Source: three-view drawing plus pictorial views. Frame: mm from the lowest corner of the part. Round coordinates to 2 decimals unless told otherwise and drop trailing zeros. Write each loop counter-clockwise with the first axis right and the second up, starting at its lowest first coordinate (ties: lowest second). Pieces come first, ordered by that corner, then holes. Notation, with made-up numbers: (20, 44) -> (45, 44) arc R23 cw to (45, 75) -> close; hole circle Ø6 at (40.25, 70). An arc over 180 degrees is marked (long way). Put each result on its own line as item: value.
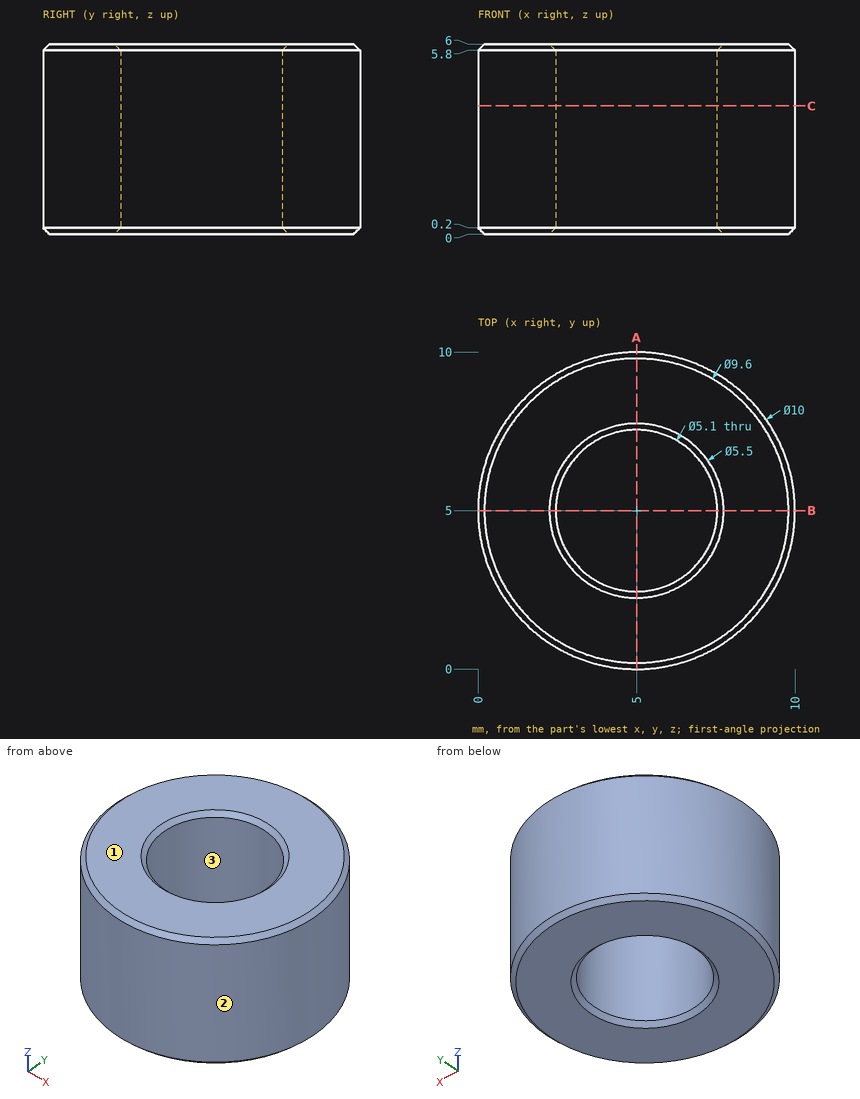
Q1. Cut plane C-C on z = 4.05. Output: boundary loops of the cut face in (x, y).
Ans:
outline: circle Ø10 at (5, 5); hole circle Ø5.1 at (5, 5)
Q2. Cut plane A-A on x = 5. Output: boundary loops of the cut face in (y, z), and give its area (3 significant figures).
Ans:
outline: (0, 0.2) -> (0.2, 0) -> (2.25, 0) -> (2.45, 0.2) -> (2.45, 5.8) -> (2.25, 6) -> (0.2, 6) -> (0, 5.8) -> close; (7.55, 0.2) -> (7.75, 0) -> (9.8, 0) -> (10, 0.2) -> (10, 5.8) -> (9.8, 6) -> (7.75, 6) -> (7.55, 5.8) -> close
area: 29.2 mm^2
Q3. Material intervals for line 1 (Y direction, x = 5, z = 4); line 2 (Y direction, x = 3.75, z = 1.2); line 3 (X direction, y = 3, z = 4.7), sorted ascending. Write a range as [from, to].
Ans:
line 1: y = [0, 2.45], [7.55, 10]
line 2: y = [0.16, 2.78], [7.22, 9.84]
line 3: x = [0.42, 3.42], [6.58, 9.58]
Q4. Draft query along X for the marked faces 1, 2 and 3. Return one class per face: +X half, -X half, draft (parallel to the pull), parting line (faces both ways), or undercut.
Ans:
face 1: draft
face 2: parting line
face 3: undercut
Q5. Pin query (flat end, axial travel): pin 1 (1 mm diameter, centred on x = 2.5, z = 5, fed in from -Y); pin 2 (2 mm diameter, centred on x = 2.5, z = 4.5, fed in from +Y). Return the tip coordinate at first contact, or that it passes through.
Ans:
pin 1: stops at y = 0.42
pin 2: stops at y = 9.77
